The listing builds one solid part. Answer for the finished solid, in the listing's coordinates (mm). A direction names the side the tool comes from. Round coordinates to 2 decimals unless told otherwise and drop trailing zeros. Order: outer loops, then holes, each group sorted by start corner. A loop starts at its lowest first (then second) coordinate and runs counter-clockwise, first axis right, second up. Notation, with made-up numbers: (-11, 69.25) - (9, 69.25) arc R25 cw to (9, 101.25) - close; hole circle Ø1 at (-38.75, 24.25). An arc over 180 degrees is marked (long way). One line per item, written item: value. Start each with the question number.
1. A tool of negligible diameter and unlimited length cuts with its end or side. For faces 5 (the flat face through (0, 0, 23)), 6 (the cylindrical face through (-17.294, -4.93, -9.133)), 7 (the flat face through (9, 0, 11)), 8 (the flat face through (0, -10, -4)), 9 (the flat face through (4, 0, -8)), from which of +Z, -Z, +X, -X, +Y, -Y can it reach the whole face along a straight path? Write none if from no direction.
2. Section A-A, the plane y = -4.5 is taken. Give the vertices of the cut face in (x, z), then the cut area to 3 significant figures.
3. Section C-C, the plane y = 4.75 is taken. Give the vertices of the cut face in (x, z), then the cut area to 3 significant figures.
4. Section D-D, the plane z = 0 is taken. Give the vertices of the cut face in (x, y).
5. For a pull along Z with two mould halves and no side action, classify faces 1 (the flat face through (-2, 10, 4)), 2 (the flat face through (0, 5, 22.266)), 3 (the flat face through (0, -5, -14.434)), 4 (the flat face through (0, 0, 0)) as released by +Z, released by -Z, zero draft, split by the parting line, or undercut.
6. Straight lines are drawn through the part: line 1 (Z direction, x = 0, y = -3); line 2 (Z direction, x = -7, y = -5.25); line 3 (Z direction, x = -12.5, y = -4). For each, find the intervals that lie inside material, in ascending order.
7. Flat-ended cylindrical pins translate along their axes: P1, Ø8, axis at y = 0, z = 7, coming from the -X side; P2, Ø0.6, axis at x = -16.5, z = -9, coming from the -Y side; P3, Ø8, axis at y = -4, z = -2.5, coming from the +X side; P4, Ø2, axis at x = -0.5, z = 19, coming from the -Y side. Find the tip coordinate at first contact, or state that the pin passes through.
8. Section B-B, the plane x = 0 is taken. Give the vertices of the cut face in (y, z).
from build123d import *

# Parameters (mm, degrees)
F1_DEPTH = 10
F3_D     = 2
F3_DEPTH = 12
F3_TIP   = 0.600860619
F4_R     = 1
F5_DEPTH = 10


with BuildPart() as f1:
    # F0 (on Front) → F1 (new body)
    with BuildSketch(Plane.XZ):
        with BuildLine():
            Line((-4.3301270189, 21.3675134595), (-20.6698729811, -6.9337567297))
            ThreePointArc((-20.6698729811, -6.9337567297), (-20.6698729811, -11.9337567297), (-16.3397459622, -14.4337567297))
            Line((-16.3397459622, -14.4337567297), (16.3397459622, -14.4337567297))
            ThreePointArc((16.3397459622, -14.4337567297), (20.6698729811, -11.9337567297), (20.6698729811, -6.9337567297))
            Line((20.6698729811, -6.9337567297), (4.3301270189, 21.3675134595))
            ThreePointArc((4.3301270189, 21.3675134595), (0, 23.8675134595), (-4.3301270189, 21.3675134595))
        make_face()
    extrude(amount=F1_DEPTH)

    # F3
    with Locations(Plane.XZ.offset(10)):
        with Locations((0, 18.8675134595), (0, 0), (16.3397459622, -9.4337567297), (-16.3397459622, -9.4337567297)):
            Hole(F3_D / 2, depth=F3_DEPTH)
            with Locations((0, 0, -(F3_DEPTH + F3_TIP / 2))):  # 118° drill point
                Cone(0, F3_D / 2, F3_TIP, mode=Mode.SUBTRACT)

    # F4 (on face) → F5 (join)
    with BuildSketch(Plane(origin=(0, 0, 0), x_dir=(-1, 0, 0), z_dir=(0, 1, 0))):
        with BuildLine():
            Line((-11.2879311067, 9.3162432703), (-17.4944465005, -1.4337567297))
            Line((-17.4944465005, -1.4337567297), (12.25, -1.4337567297))
            Line((12.25, -1.4337567297), (12.25, -14.4337567297))
            Line((12.25, -14.4337567297), (16.3397459622, -14.4337567297))
            ThreePointArc((16.3397459622, -14.4337567297), (20.6698729811, -11.9337567297), (20.6698729811, -6.9337567297))
            Line((20.6698729811, -6.9337567297), (4.3301270189, 21.3675134595))
            ThreePointArc((4.3301270189, 21.3675134595), (4.0238527859, 21.8354435053), (3.6672381533, 22.2662432703))
            Line((3.6672381533, 22.2662432703), (-3.6672381533, 22.2662432703))
            ThreePointArc((-3.6672381533, 22.2662432703), (-4.0238527859, 21.8354435053), (-4.3301270189, 21.3675134595))
            Line((-4.3301270189, 21.3675134595), (-8.65, 13.885273974))
            Line((-8.65, 13.885273974), (-8.65, 9.3162432703))
            Line((-8.65, 9.3162432703), (-11.2879311067, 9.3162432703))
        make_face()
        with Locations((16.3397459622, -9.4337567297)):
            Circle(F4_R, mode=Mode.SUBTRACT)
        Circle(F4_R, mode=Mode.SUBTRACT)
        with Locations((0, 18.8675134595)):
            Circle(F4_R, mode=Mode.SUBTRACT)
        with Locations((16.3397459622, -9.4337567297)):
            Circle(F4_R)
        Circle(F4_R)
        with Locations((0, 18.8675134595)):
            Circle(F4_R)
    extrude(amount=F5_DEPTH)


solid = f1.part
Answer list:
1. face 5: +Z, +X, -X, +Y
1. face 6: -Y
1. face 7: +Z, +X, +Y
1. face 8: +Z, -Z, +X, -X, -Y
1. face 9: -Z, +X, +Y
2. outline: (-20.67, -6.93) arc R5 ccw to (-16.34, -14.43) - (16.34, -14.43) arc R5 ccw to (20.67, -6.93) - (4.33, 21.37) arc R5 ccw to (-4.33, 21.37) - close; hole circle Ø2 at (-16.34, -9.43); hole circle Ø2 at (0, 0); hole circle Ø2 at (0, 18.87); hole circle Ø2 at (16.34, -9.43)
2. area: 1,020 mm²
3. outline: (-20.67, -6.93) arc R5 ccw to (-16.34, -14.43) - (-12.25, -14.43) - (-12.25, -1.43) - (17.49, -1.43) - (11.29, 9.32) - (8.65, 9.32) - (8.65, 13.89) - (4.33, 21.37) arc R5 ccw to (3.67, 22.27) - (-3.67, 22.27) arc R5 ccw to (-4.33, 21.37) - close
3. area: 599 mm²
4. outline: (-16.67, -10) - (-1, -10) - (-1, 0) - (1, 0) - (1, -10) - (16.67, -10) - (16.67, 10) - (-16.67, 10) - close
5. face 1: zero draft
5. face 2: released by +Z
5. face 3: released by -Z
5. face 4: undercut
6. line 1: z = -14.43 to -1, 1 to 17.87, 19.87 to 23.87
6. line 2: z = -14.43 to 16.74
6. line 3: z = -14.43 to 7.22
7. P1: stops at x = -14.93
7. P2: stops at y = 0
7. P3: stops at x = 20.42
7. P4: stops at y = -10
8. outline: (-10, -14.43) - (0, -14.43) - (0, -1.43) - (10, -1.43) - (10, 22.27) - (0, 22.27) - (0, 23.87) - (-10, 23.87) - (-10, 19.87) - (0, 19.87) - (0, 17.87) - (-10, 17.87) - (-10, 1) - (0, 1) - (0, -1) - (-10, -1) - close
